from build123d import *

# Parameters (mm, degrees)
SKETCH_1_W          = 190
SKETCH_1_H          = 40
EXTRUDE_1_DEPTH     = 2
CUT_EXTRUDE_1_DEPTH = 2
SKETCH_3_R          = 2.05
CUT_EXTRUDE_2_DEPTH = 2
FILLET_1_R          = 3


with BuildPart() as part:
    # 草图1 → 凸台-拉伸1 (new body)
    with BuildSketch(Plane.XY):
        Rectangle(SKETCH_1_W, SKETCH_1_H)
    extrude(amount=EXTRUDE_1_DEPTH)

    # 草图2 → 切除-拉伸1 (cut)
    with BuildSketch(Plane.XY.offset(2)):
        with BuildLine():
            Line((0, -5), (0, 20))
            Line((0, 20), (-80, 20))
            ThreePointArc((-80, 20), (-72.67766953, 2.32233047), (-55, -5))
            Line((-55, -5), (0, -5))
        make_face()
        with BuildLine():
            Line((80, 20), (0, 20))
            Line((0, 20), (0, -5))
            Line((0, -5), (55, -5))
            ThreePointArc((55, -5), (72.67766953, 2.32233047), (80, 20))
        make_face()
    extrude(amount=-CUT_EXTRUDE_1_DEPTH, mode=Mode.SUBTRACT)

    # 草图3 → 切除-拉伸2 (cut)
    with BuildSketch(Plane.XY.offset(2)):
        with Locations((-87.5, 15)):
            Circle(SKETCH_3_R)
        with Locations((-87.5, -15)):
            Circle(SKETCH_3_R)
        with Locations(Location((87.5, -15, 0), (0, 0, 180))):
            Circle(SKETCH_3_R)
        with Locations(Location((87.5, 15, 0), (0, 0, 180))):
            Circle(SKETCH_3_R)
    extrude(amount=-CUT_EXTRUDE_2_DEPTH, mode=Mode.SUBTRACT)

    # 圆角1
    fillet_1_edges = [part.edges().sort_by_distance(p)[0] for p in [
        (-80, 20, 1),
        (80, 20, 1),
        (95, -20, 1),
        (-95, -20, 1),
        (-95, 20, 1),
        (95, 20, 1),
    ]]
    fillet(fillet_1_edges, radius=FILLET_1_R)


solid = part.part
Input: part model. Units: mm. Frame: model coordinates. A direction names the side the tool comes from. Give positions to 0.01 mm unless a question says otherwise; leave off trailing zeros. Loops run counter-clockwise (first coordinate to the right, second up) from the corner with the lowest first, then second, coordinate; pieces in that order, holes last. Notation, with made-up numbers: (45, -32) - (69, -32) arc R21 cw to (69, -27) - close; hole circle Ø3 at (10.5, -29.75). An arc over 180 degrees is marked (long way). Use CSV: the item, a comma, the result in double quotes. Start each with the question number.
Item 1: Section A-A on x = -87.5. Return loops of the section in (y, z).
Item 2: Section D-D on y = 6.5. Return loops of the section in (x, z), then the cut area to 3 significant figures.
Item 3: Reachability of faces 1 (the cylindrical face through (-71.89, 1.57, 1.01)), 2 (the cylindrical face through (94.1, -19.14, 1.01)) from +Z, -Z, +X, -X, +Y, -Y: full face, straight path, thin tool, end or side. Return the list, or none.
Item 4: Section B-B on y = -15. Return loops of the section in (x, z), then the cut area to 3 significant figures.
Item 5: Line query: line 1 (Y direction, x = -87.5, z = 0.55); line 2 (X direction, y = -16.5, z = 1.85); line 3 (Y direction, x = 29, z = 1.45). Output: solid intervals per line, ascending.
Item 6: Section C-C on z = 0.6. Return loops of the section in (x, y).
Item 7: Mould query, pull axis X, two halves, no side actions, for faces 3 (the cylindrical face through (94.14, 19.1, 1.01)), 4 (the cylindrical face through (89.55, 14.91, 1.01)), 5 (the cylindrical face through (-94.14, 19.1, 1.01)). Classes: pulls with the +X half, pulls with the -X half, needs draft (parallel to the pull), parting line crosses it, or undercut.
Item 8: Contact query for a flat-ended pin moving along its axis: P1, Ø0.6, axis at x = -25.5, z = 1, coming from the +Y side. Output: stop coordinate, or through.
Ans:
1,outline,"(-20, 0) - (-17.05, 0) - (-17.05, 2) - (-20, 2) - close; (-12.95, 0) - (12.95, 0) - (12.95, 2) - (-12.95, 2) - close; (17.05, 0) - (20, 0) - (20, 2) - (17.05, 2) - close"
2,outline,"(-95, 0) - (-76.04, 0) - (-76.04, 2) - (-95, 2) - close; (76.04, 0) - (95, 0) - (95, 2) - (76.04, 2) - close"
2,area,"75.8 mm2"
3,face 1,"+Z, -Z, +Y"
3,face 2,"+Z, -Z, +X, -Y"
4,outline,"(-95, 0) - (-89.55, 0) - (-89.55, 2) - (-95, 2) - close; (-85.45, 0) - (85.45, 0) - (85.45, 2) - (-85.45, 2) - close; (89.55, 0) - (95, 0) - (95, 2) - (89.55, 2) - close"
4,area,"364 mm2"
5,line 1,"y = -20 to -17.05, -12.95 to 12.95, 17.05 to 20"
5,line 2,"x = -95 to -88.9, -86.1 to 86.1, 88.9 to 95"
5,line 3,"y = -20 to -5"
6,outline,"(-95, -17) arc R3 ccw to (-92, -20) - (92, -20) arc R3 ccw to (95, -17) - (95, 17) arc R3 ccw to (92, 20) - (82.84, 20) arc R3 ccw to (79.86, 17.32) arc R25 cw to (55, -5) - (-55, -5) arc R25 cw to (-79.86, 17.32) arc R3 ccw to (-82.84, 20) - (-92, 20) arc R3 ccw to (-95, 17) - close; hole circle Ø4.1 at (-87.5, -15); hole circle Ø4.1 at (-87.5, 15); hole circle Ø4.1 at (87.5, -15); hole circle Ø4.1 at (87.5, 15)"
7,face 3,"pulls with the +X half"
7,face 4,"undercut"
7,face 5,"pulls with the -X half"
8,P1,"stops at y = -5"
